Geometry check sheet. Reference: the model listing, model coordinates, mm. A direction names the side the tool comes from. Give positions to 0.01 mm unless a question says otherwise; leave off trailing zeros. Loops run counter-clockwise (first coordinate to the right, second up) from the corner with the lowest first, then second, coordinate; pieces in that order, holes last. Notation, with made-up numbers: (56, 74) -> (75, 74) arc R25 cw to (75, 109) -> close; hole circle Ø5 at (19.25, 63). An arc over 180 degrees is marked (long way). Answer as a JSON object with one key per item and string values.
from build123d import *

# Parameters (mm, degrees)
SKETCH1_W           = 57.15
SKETCH1_H           = 31.75
SKETCH1_W_2         = 50.8
SKETCH1_H_2         = 25.4
BOSS_EXTRUDE1_DEPTH = 406.4
SKETCH2_R           = 2.5
CUT_EXTRUDE1_DEPTH  = 409.638658383


with BuildPart() as part:
    # Sketch1 → Boss-Extrude1 (new body)
    with BuildSketch(Plane(origin=(0, 0, 0), x_dir=(1, 0, 0), z_dir=(0, 1, 0))):
        Rectangle(SKETCH1_W, SKETCH1_H)
        Rectangle(SKETCH1_W_2, SKETCH1_H_2, mode=Mode.SUBTRACT)
    extrude(amount=BOSS_EXTRUDE1_DEPTH)

    # Sketch2 → Cut-Extrude1 (cut, through all)
    with BuildSketch(Plane.XY.offset(15.875)):
        with Locations((-11.25, 60)):
            Circle(SKETCH2_R)
        with Locations((-11.25, 25)):
            Circle(SKETCH2_R)
        with Locations((11.25, 25)):
            Circle(SKETCH2_R)
        with Locations((11.25, 60)):
            Circle(SKETCH2_R)
    cut_extrude1 = extrude(amount=-CUT_EXTRUDE1_DEPTH, mode=Mode.SUBTRACT)

    # Mirror1: Cut-Extrude1 across plane
    add(cut_extrude1.mirror(Plane(origin=(0, 203.2, 0), x_dir=(0, 0, 1), z_dir=(0, -1, 0))), mode=Mode.SUBTRACT)


solid = part.part
1) Draft check along X on faces 1 (the face through (0, 200, 12.7)), 2 (the face through (0, 200, -15.875)), 3 (the face through (25.4, 200, 0)), 4 (the face through (28.575, 200, 0)). Enter one of: pulls with the +X half, pulls with the -X half, needs draft (parallel to the pull), parting line crosses it, or undercut.
Geometry check:
{"face 1": "undercut", "face 2": "needs draft", "face 3": "undercut", "face 4": "pulls with the +X half"}
2) Section check A-A on z = 8. Record the cut outline in (x, y) (3 decimals), plus the area to 3 significant figures.
Geometry check:
{"outline": "(-28.575, 0) -> (-25.4, 0) -> (-25.4, 406.4) -> (-28.575, 406.4) -> close; (25.4, 0) -> (28.575, 0) -> (28.575, 406.4) -> (25.4, 406.4) -> close", "area": "2,580 mm2"}
3) Material ranges on line 1 along X through (y, z) = (346.4, -13.45) (3 decimals); line 2 along Y through (x, z) = (-11.25, 15.1); line 3 along Z through (x, y) = (6, 295) (3 decimals), recorded low to high. Write a range as from..to.
Geometry check:
{"line 1": "x = -28.575..-13.75, -8.75..8.75, 13.75..28.575", "line 2": "y = 0..22.5, 27.5..57.5, 62.5..343.9, 348.9..378.9, 383.9..406.4", "line 3": "z = -15.875..-12.7, 12.7..15.875"}
4) Section check B-B on y = 207.5. Record the cut outline in (x, z) (3 decimals).
Geometry check:
{"outline": "(-28.575, -15.875) -> (28.575, -15.875) -> (28.575, 15.875) -> (-28.575, 15.875) -> close; hole (-25.4, -12.7) -> (25.4, -12.7) -> (25.4, 12.7) -> (-25.4, 12.7) -> close"}
5) Tool access check on faces 5 (the face through (0, 200, -12.7)), 6 (the face through (-4, 0, 13)). Record the directions out of +Z, -Z, +X, -X, +Y, -Y that give a thin tool (end or side, any length) a straight path to the whole face; none if there is none.
Geometry check:
{"face 5": "+Y, -Y", "face 6": "+Z, -Z, +X, -X, -Y"}
